Can you work these out from the model? Positions are in its coordinate system, mm. A direction names the side the tool comes from. Give positions to 0.01 mm unless a question says otherwise; leave off trailing zeros. Loops run counter-clockwise (first coordinate to the right, second up) from the corner with the lowest first, then second, coordinate; pieces in that order, holes last.
from build123d import *

# Parameters (mm, degrees)
F0_W      = 42.3
F0_H      = 42.3
F0_R      = 1.75
F0_R_2    = 3
F1_DEPTH  = 3
F2_R      = 11.5
F3_DEPTH  = 2
F4_R      = 1.75
F5_DEPTH  = 16
F9_W      = 15
F9_H      = 11
F10_DEPTH = 19
F11_DEPTH = 10
F18_DEPTH = 11.251
F19_W     = 28.3221583813
F19_H     = 99.7033566236
F20_DEPTH = 22.051
F22_DEPTH = 16.0051434669
F23_R     = 2.75
F23_R_2   = 1.75
F24_DEPTH = 1


# Not quite as in the source:
# - a feature names something its author has since deleted; it is built from what else it names


with BuildPart() as f1:
    # F0 (on Front) → F1 (new body)
    with BuildSketch(Plane.XZ):
        Rectangle(F0_W, F0_H)
        with Locations((-15.5, -15.5)):
            Circle(F0_R, mode=Mode.SUBTRACT)
        with Locations((-15.5, 15.5)):
            Circle(F0_R, mode=Mode.SUBTRACT)
        Circle(F0_R_2, mode=Mode.SUBTRACT)
        with Locations((15.5, 15.5)):
            Circle(F0_R, mode=Mode.SUBTRACT)
    extrude(amount=F1_DEPTH)

    # F2 (on face) → F3 (cut)
    with BuildSketch(Plane(origin=(0, 0, 0), x_dir=(-1, 0, 0), z_dir=(0, 1, 0))):
        Circle(F2_R)
    extrude(amount=-F3_DEPTH, mode=Mode.SUBTRACT)

    # F4 (on face) → F5 (join)
    with BuildSketch(Plane.XZ.offset(3)):
        with BuildLine():
            Line((-11.75, 21.15), (-21.15, 21.15))
            Line((-21.15, 21.15), (-21.15, -21.15))
            Line((-21.15, -21.15), (21.15, -21.15))
            Line((21.15, -21.15), (21.15, -18.15))
            Line((21.15, -18.15), (-12.8467001677, -18.15))
            ThreePointArc((-12.8467001677, -18.15), (-12.8483495706, -12.8483495706), (-18.15, -12.8467001677))
            Line((-18.15, -12.8467001677), (-18.15, 12.8467001677))
            ThreePointArc((-18.15, 12.8467001677), (-14.0638593384, 12.0358983849), (-11.75, 15.5))
            Line((-11.75, 15.5), (-11.75, 21.15))
        make_face()
        with Locations((-15.5, -15.5)):
            Circle(F4_R, mode=Mode.SUBTRACT)
        with Locations((-15.5, 15.5)):
            Circle(F4_R, mode=Mode.SUBTRACT)
    extrude(amount=F5_DEPTH)

    # F9 (on Front) → F10 (join, through all)
    with BuildSketch(Plane.XZ):
        with Locations((-13.65, 25)):
            Rectangle(F9_W, F9_H)
    extrude(amount=F10_DEPTH)

    # F8 (on offset) → F11 (cut)
    with BuildSketch(Plane.XZ.offset(9.65)):
        Polygon((0, 22), (0, 28), (-18.65, 28), (-18.65, 28.5), (-20.15, 28.5), (-21.15, 27), (-21.15, 23), (-20.15, 21.5), (-18.65, 21.5), (-18.65, 22), align=None)
    extrude(amount=F11_DEPTH, mode=Mode.SUBTRACT)

    # F13 (on offset) → F14 (revolve, cut)
    with BuildSketch(Plane.XZ.offset(9.65)):
        Polygon((17.05, -18.15), (19.05, -18.15), (19.05, -12.65), (10.8, -12.65), (10.8, -26.95), (19.05, -26.95), (19.05, -22.35), (17.05, -22.35), align=None)
    revolve(axis=Axis((10.8, -9.65, -5.160998553), (0, 0, -1)), mode=Mode.SUBTRACT)

    # F15 (on offset) → F16 (revolve)
    with BuildSketch(Plane.XZ.offset(9.65)):
        Polygon((19.05, -18.15), (17.05, -18.15), (17.05, -22.35), (19.05, -22.35), (19.05, -26.95), (22.05, -26.95), (22.05, -18.15), align=None)
    revolve(axis=Axis((10.8, -9.65, -5.160998553), (0, 0, -1)))

    # F17 (on offset) → F18 (cut, through all)
    with BuildSketch(Plane.XZ.offset(9.65)):
        Polygon((2.55, -12.65), (2.55, -18.15), (4.55, -18.15), (4.55, -22.35), (2.55, -22.35), (2.55, -26.95), (19.05, -26.95), (19.05, -22.35), (17.05, -22.35), (17.05, -18.15), (19.05, -18.15), (19.05, -12.65), align=None)
    extrude(amount=F18_DEPTH, mode=Mode.SUBTRACT)

    # F19 (on Right) → F20 (cut, through all)
    with BuildSketch(Plane.YZ):
        with Locations((14.1610791907, -2.7998201549)):
            Rectangle(F19_W, F19_H)
    extrude(amount=F20_DEPTH, mode=Mode.SUBTRACT)

    # F21 (on face) → F22 (cut, through all)
    with BuildSketch(Plane.XZ.offset(3)):
        with BuildLine():
            ThreePointArc((-4.9008020267, -0.9910295129), (0.9910295129, -4.9008020267), (4.9008020267, 0.9910295129))
            Line((4.9008020267, 0.9910295129), (-4.0184635896, 45.0982477529))
            ThreePointArc((-4.0184635896, 45.0982477529), (-9.9102951291, 49.0080202666), (-13.8200676429, 43.116188727))
            Line((-13.8200676429, 43.116188727), (-4.9008020267, -0.9910295129))
        make_face()
    extrude(amount=F22_DEPTH, mode=Mode.SUBTRACT)

    # F23 (on face) → F24 (cut)
    with BuildSketch(Plane.XZ.offset(3)):
        with Locations((15.5, 15.5)):
            Circle(F23_R)
        with Locations((15.5, 15.5)):
            Circle(F23_R_2, mode=Mode.SUBTRACT)
    extrude(amount=-F24_DEPTH, mode=Mode.SUBTRACT)


solid = f1.part
(1) Will these pins go through, and if not, where does the flat tip stop? P1, Ø3.5, axis at x = 20, y = -3, coming from the -Z side; P2, Ø4, axis at y = -3, z = -17.5, coming from the +X side; P3, Ø4, axis at x = 17, z = -3, coming from the -Y side; P4, Ø9, axis at x = 9, y = -7, coming from the +Z side.
Returned:
P1: stops at z = -26.95
P2: stops at x = 21.15
P3: stops at y = -3
P4: stops at z = 21.15
(2) Suppose I cut it at B-B on x = -15.5. List the corners of the cut face in (y, z) for me.
Returned:
outline: (-19, -21.15) - (0, -21.15) - (0, -17.25) - (-19, -17.25) - close; (-19, -13.75) - (0, -13.75) - (0, 13.75) - (-19, 13.75) - (-19, 11.75) - (-3, 11.75) - (-3, -11.75) - (-19, -11.75) - close; (-19, 17.25) - (0, 17.25) - (0, 30.5) - (-19, 30.5) - (-19, 28) - (-9.65, 28) - (-9.65, 22) - (-19, 22) - close
(3) Please list where these lines run through material, in increasing order: probe 1 along Z at (x, y) = (-15.5, -10.5); probe 2 along Z at (x, y) = (0, -2.7); probe 3 along Z at (x, y) = (15.5, -2.4).
Returned:
probe 1: z = -21.15 to -17.25, -13.75 to -11.75, 11.75 to 13.75, 17.25 to 22, 28 to 30.5
probe 2: z = -21.15 to -3, 3 to 21.15
probe 3: z = -26.95 to 12.75, 18.25 to 21.15
(4) Suppose I cut it at D-D on z = 10.5. List the corners of the cut face in (x, y) for me, plus the area to 3 significant figures.
Returned:
outline: (-21.15, -19) - (-18.15, -19) - (-18.15, -3) - (21.15, -3) - (21.15, 0) - (4.69, 0) - (4.69, -2) - (-4.69, -2) - (-4.69, 0) - (-21.15, 0) - close
area: 156 mm2
(5) Suppose I cut it at A-A on z = -15.5. List the corners of the cut face in (x, y) for me, plus the area to 3 significant figures.
Returned:
outline: (-21.15, -19) - (-17.25, -19) - (-17.25, 0) - (-21.15, 0) - close; (-13.75, -19) - (-11.75, -19) - (-11.75, -3) - (5.92, -3) arc R8.25 cw to (15.68, -3) - (21.15, -3) - (21.15, 0) - (-13.75, 0) - close
area: 200 mm2
(6) Suppose I cut it at C-C on y = -7. List the corners of the cut face in (x, z) for me.
Returned:
outline: (-21.15, -21.15) - (-0.13, -21.15) - (-0.13, -26.95) - (2.99, -26.95) - (2.99, -22.35) - (5.14, -22.35) - (5.14, -18.15) - (-12.85, -18.15) arc R3.75 ccw to (-18.15, -12.85) - (-18.15, 12.85) arc R3.75 ccw to (-11.75, 15.5) - (-11.75, 19.5) - (-9.04, 19.5) - (-11.27, 30.5) - (-21.15, 30.5) - close; (16.46, -22.35) - (18.61, -22.35) - (18.61, -26.95) - (21.73, -26.95) - (21.73, -18.15) - (16.46, -18.15) - close; hole circle Ø3.5 at (-15.5, -15.5); hole circle Ø3.5 at (-15.5, 15.5)
(7) Thinking about a two-plate mould opening in X: for faces 1 (the cylindrical face through (22.04, -9.22, -23.47)), 2 (the flat face through (-15, -9, 30.5)), 3 (the cylindrical face through (-14.6, -9.4, -14)), which applies, pulls with the +X half, pulls with the -X half, needs draft (parallel to the pull), parting line crosses it, or undercut?
Returned:
face 1: pulls with the +X half
face 2: needs draft
face 3: undercut
(8) Which directions (+Z, -Z, +X, -X, +Y, -Y) give clear straight access to the entire face, cutting with the end or side of a thin tool? Please do faces 4 (the cylindrical face through (10.7, -1.4, -15.4)), 5 (the flat face through (-6.15, -1, 26)), 6 (the flat face through (17.05, -14, -20)), 7 (the flat face through (-10.172, -9.11, 25.077)).
Returned:
face 4: -Y
face 5: +Z, +X, +Y, -Y
face 6: +Z, -Z, -Y
face 7: +Z, +X, -Y
